from build123d import *

# Parameters (mm, degrees)
CROQUIS1_W              = 23
CROQUIS1_H              = 23
SALIENTE_EXTRUIR4_DEPTH = 10
CROQUIS2_W              = 2
CROQUIS2_H              = 8.5
CORTAR_EXTRUIR2_DEPTH   = 28.590759323
CORTAR_EXTRUIR6_DEPTH   = 28.590759323
REDONDEO14_R            = 0.5
REDONDEO15_R            = 0.5


with BuildPart() as part:
    # Croquis1 → Saliente-Extruir4 (new body)
    with BuildSketch(Plane(origin=(0, 0, 0), x_dir=(1, 0, 0), z_dir=(0, 1, 0))):
        Rectangle(CROQUIS1_W, CROQUIS1_H)
    extrude(amount=SALIENTE_EXTRUIR4_DEPTH)

    # Croquis2 → Cortar-Extruir2 (cut, through all)
    with BuildSketch(Plane.XY.offset(11.5)):
        with Locations((-7.5, 5.75)):
            Rectangle(CROQUIS2_W, CROQUIS2_H)
        with Locations((-2.5, 5.75)):
            Rectangle(CROQUIS2_W, CROQUIS2_H)
        with Locations((2.5, 5.75)):
            Rectangle(CROQUIS2_W, CROQUIS2_H)
        with Locations((7.5, 5.75)):
            Rectangle(CROQUIS2_W, CROQUIS2_H)
    extrude(amount=-CORTAR_EXTRUIR2_DEPTH, mode=Mode.SUBTRACT)

    # Croquis3 → Cortar-Extruir6 (cut, through all)
    with BuildSketch(Plane(origin=(11.5, 0, 0), x_dir=(0, 0, -1), z_dir=(1, 0, 0))):
        with BuildLine():
            Line((-10.5, 10), (-7.1, 10))
            Line((-7.1, 10), (-7.1, 3.7))
            ThreePointArc((-7.1, 3.7), (-8.8, 2), (-10.5, 3.7))
            Line((-10.5, 3.7), (-10.5, 10))
        make_face()
        with BuildLine():
            Line((-6.1, 10), (-6.1, 3.7))
            ThreePointArc((-6.1, 3.7), (-4.4, 2), (-2.7, 3.7))
            Line((-2.7, 3.7), (-2.7, 10))
            Line((-2.7, 10), (-6.1, 10))
        make_face()
        with BuildLine():
            Line((-1.7, 10), (-1.7, 3.7))
            ThreePointArc((-1.7, 3.7), (0, 2), (1.7, 3.7))
            Line((1.7, 3.7), (1.7, 10))
            Line((1.7, 10), (-1.7, 10))
        make_face()
        with BuildLine():
            Line((2.7, 10), (2.7, 3.7))
            ThreePointArc((2.7, 3.7), (4.4, 2), (6.1, 3.7))
            Line((6.1, 3.7), (6.1, 10))
            Line((6.1, 10), (2.7, 10))
        make_face()
        with BuildLine():
            Line((7.1, 10), (7.1, 3.7))
            ThreePointArc((7.1, 3.7), (8.8, 2), (10.5, 3.7))
            Line((10.5, 3.7), (10.5, 10))
            Line((10.5, 10), (7.1, 10))
        make_face()
    extrude(amount=-CORTAR_EXTRUIR6_DEPTH, mode=Mode.SUBTRACT)

    # Redondeo14
    redondeo14_edges = [part.edges().sort_by_distance(p)[0] for p in [
        (-5, 10, -2.7),
        (-5, 10, -1.7),
        (-10, 10, -2.7),
        (-10, 10, -1.7),
        (-10, 10, 1.7),
        (-10, 10, 2.7),
        (-5, 10, 1.7),
        (-5, 10, 2.7),
        (-5, 10, 6.1),
        (-5, 10, 7.1),
        (-5, 10, 10.5),
        (-5, 10, 11.5),
        (-10, 10, 6.1),
        (-10, 10, 7.1),
        (-10, 10, 10.5),
        (-10, 10, 11.5),
        (0, 10, -2.7),
        (0, 10, -1.7),
        (0, 10, 1.7),
        (0, 10, 2.7),
        (0, 10, 6.1),
        (0, 10, 7.1),
        (0, 10, 10.5),
        (0, 10, 11.5),
        (5, 10, 11.5),
        (5, 10, 10.5),
        (5, 10, 7.1),
        (5, 10, 6.1),
        (5, 10, 2.7),
        (5, 10, 1.7),
        (5, 10, -1.7),
        (5, 10, -2.7),
        (5, 10, -6.1),
        (5, 10, -7.1),
        (0, 10, -6.1),
        (0, 10, -7.1),
        (-5, 10, -6.1),
        (-5, 10, -7.1),
        (-10, 10, -6.1),
        (-10, 10, -7.1),
        (-10, 10, -10.5),
        (-10, 10, -11.5),
        (-5, 10, -10.5),
        (-5, 10, -11.5),
        (0, 10, -11.5),
        (5, 10, -11.5),
        (10, 10, 10.5),
        (10, 10, 11.5),
        (10, 10, 7.1),
        (10, 10, 6.1),
        (10, 10, 2.7),
        (10, 10, 1.7),
        (10, 10, -1.7),
        (10, 10, -2.7),
        (10, 10, -7.1),
        (10, 10, -6.1),
        (10, 10, -10.5),
        (10, 10, -11.5),
    ]]
    fillet(redondeo14_edges, radius=REDONDEO14_R - 0.0001)  # a hair under: the kernel refuses the full size

    # Redondeo15
    redondeo15_edges = [part.edges().sort_by_distance(p)[0] for p in [
        (5, 10, -10.5),
        (0, 10, -10.5),
    ]]
    fillet(redondeo15_edges, radius=REDONDEO15_R)


solid = part.part
Could you check a few things on this model? Use its own coordinates, in mm. A direction names the side the tool comes from. Give positions to 0.01 mm unless a question says otherwise; leave off trailing zeros. Order: outer loops, then holes, each group sorted by start corner. A loop starts at its lowest first (then second) coordinate and runs counter-clockwise, first axis right, second up. Notation, with made-up numbers: (6.5, 32) - (62.5, 32) arc R31 cw to (62.5, 67) - close; hole circle Ø7 at (34.25, 18.5). An arc over 180 degrees is marked (long way). One line per item, written item: value. Start each with the question number.
1. Imagine slicing it at B-B on x = -7.25. List the corners of the cut face in (y, z) for me.
2. Thinking about a two-plate mould opening in Z: for faces 4 (the face through (-5, 2, -4.4)), 5 (the face through (-1.5, 5, 2)), which applies, +Z half, -Z half, draft (parallel to the pull), parting line (faces both ways), or undercut?
3. If I drill on probe 1 along X at (y, z) = (5.5, -7); probe 2 along Z at (x, y) = (9.5, 7); probe 3 along Z at (x, y) = (-4.5, 2.75), over which ranges is the centre line in solid material (lowest first)?
4. For P1, Ø2, axis at x = 7, z = 5, coming from the +Y side; P2, Ø0.6, axis at x = 2.5, z = 0.5, coming from the +Y side, each with a flat end and sliding along its axis, tell me the tip position at first contact or that it passes through.
5. Imagine slicing it at C-C on y = 6. Give the number of separate pieces and of enclosed holes in the cut face, plus the area to 3 significant figures.
6. For faces 1 (the face through (7, 1.5, 0)), 2 (the face through (0, 7, 7.1)), 3 (the face through (0, 0, 0)), which set-ups out of +Z, -Z, +X, -X, +Y, -Y let a thin tool reach every point of the face, with its end or its side?
7. Imagine slicing it at A-A on z = -4.4. List the corners of the cut face in (x, y) for me.
8. Imagine slicing it at D-D on z = 3. List the corners of the cut face in (x, y) for me, plus the area to 3 significant figures.
Values:
1. outline: (0, -11.5) - (1.5, -11.5) - (1.5, 11.5) - (0, 11.5) - close
2. face 4: undercut
2. face 5: draft
3. probe 1: -11.5 to -8.5, -6.5 to -3.5, -1.5 to 1.5, 3.5 to 6.5, 8.5 to 11.5
3. probe 2: -11.5 to -10.5, -7.1 to -6.1, -2.7 to -1.7, 1.7 to 2.7, 6.1 to 7.1, 10.5 to 11.5
3. probe 3: -11.5 to -10.21, -7.39 to -5.81, -2.99 to -1.41, 1.41 to 2.99, 5.81 to 7.39, 10.21 to 11.5
4. P1: y = 2.84
4. P2: y = 1.5
5. separate pieces: 30
5. enclosed holes: 0
5. area: 90.0 mm²
6. face 1: +Z, -Z, +Y
6. face 2: +X, -X, +Y
6. face 3: +Z, -Z, +X, -X, -Y
7. outline: (-11.5, 0) - (11.5, 0) - (11.5, 2) - (8.5, 2) - (8.5, 1.5) - (6.5, 1.5) - (6.5, 2) - (3.5, 2) - (3.5, 1.5) - (1.5, 1.5) - (1.5, 2) - (-1.5, 2) - (-1.5, 1.5) - (-3.5, 1.5) - (-3.5, 2) - (-6.5, 2) - (-6.5, 1.5) - (-8.5, 1.5) - (-8.5, 2) - (-11.5, 2) - close
8. outline: (-11.5, 0) - (11.5, 0) - (11.5, 2.74) - (8.5, 2.74) - (8.5, 1.5) - (6.5, 1.5) - (6.5, 2.74) - (3.5, 2.74) - (3.5, 1.5) - (1.5, 1.5) - (1.5, 2.74) - (-1.5, 2.74) - (-1.5, 1.5) - (-3.5, 1.5) - (-3.5, 2.74) - (-6.5, 2.74) - (-6.5, 1.5) - (-8.5, 1.5) - (-8.5, 2.74) - (-11.5, 2.74) - close
8. area: 53.0 mm²
